Can you work these out from the model? Positions are in its coordinate system, mm. Coordinates: 2 decimals unless noted, no trailing zeros. Loops run counter-clockwise (first coordinate to the right, second up) from the corner with the lowest first, then second, coordinate; pieces in that order, holes last. Notation, with made-up numbers: (82.25, 61) -> (88.25, 61) arc R10 ccw to (88.25, 79) -> close; hole circle Ø2 at (68, 22.25). An arc over 180 degrees is marked (long way). Use one line per item in the form item = value. Start each with the question number.
(1) Imagine slicing it at C-C (y = -24.5). List the corners of the cut face in (x, z) for me.
(2) Imagine slicing it at B-B (z = 8.25). List the corners of the cut face in (x, y) for me.
(3) Imagine slicing it at A-A (x = -3.5). List the corners of the cut face in (y, z) for me.
(4) I need wall thicknesses on line 1 (X direction, y = -22.95, z = 15.5); line 2 (Z direction, x = -44.5, y = -23); line 3 (Z direction, x = -3.5, y = -24.65). Which ranges of each line are inside material? Lowest first, please. Write a range as [from, to].
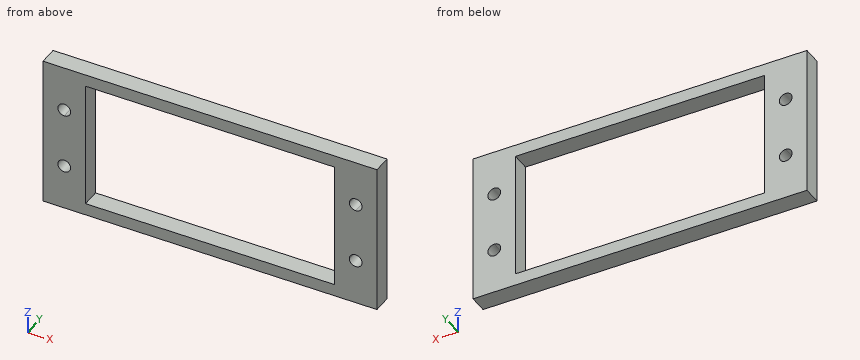
```python
from build123d import *

# Parameters (mm, degrees)
F1_START = 22
F0_W     = 55
F0_H     = 25
F1_DEPTH = 3


with BuildPart() as f1:
    # F0 (on Front) → F1 (new body)
    with BuildSketch(Plane.XZ.offset(F1_START)):
        with Locations((-20.5, 10.5)):
            Rectangle(F0_W, F0_H)
        with BuildLine():
            Line((0, 5.5), (0, 0))
            Line((0, 0), (-41, 0))
            Line((-41, 0), (-41, 5.5))
            Line((-41, 5.5), (-43.45, 5.5))
            ThreePointArc((-43.45, 5.5), (-45.2424621202, 4.7575378798), (-44.5, 6.55))
            Line((-44.5, 6.55), (-44.5, 14.45))
            ThreePointArc((-44.5, 14.45), (-45.2424621202, 16.2424621202), (-43.45, 15.5))
            Line((-43.45, 15.5), (-41, 15.5))
            Line((-41, 15.5), (-41, 21))
            Line((-41, 21), (0, 21))
            Line((0, 21), (0, 15.5))
            Line((0, 15.5), (2.45, 15.5))
            ThreePointArc((2.45, 15.5), (3.5, 16.55), (4.55, 15.5))
            ThreePointArc((4.55, 15.5), (4.2424621202, 14.7575378798), (3.5, 14.45))
            Line((3.5, 14.45), (3.5, 6.55))
            ThreePointArc((3.5, 6.55), (4.2424621202, 6.2424621202), (4.55, 5.5))
            ThreePointArc((4.55, 5.5), (3.5, 4.45), (2.45, 5.5))
            Line((2.45, 5.5), (0, 5.5))
        make_face(mode=Mode.SUBTRACT)
        with BuildLine():
            Line((-43.45, 5.5), (-41, 5.5))
            Line((-41, 5.5), (-41, 15.5))
            Line((-41, 15.5), (-43.45, 15.5))
            ThreePointArc((-43.45, 15.5), (-43.7575378798, 14.7575378798), (-44.5, 14.45))
            Line((-44.5, 14.45), (-44.5, 6.55))
            ThreePointArc((-44.5, 6.55), (-43.7575378798, 6.2424621202), (-43.45, 5.5))
        make_face()
        with BuildLine():
            Line((0, 15.5), (0, 5.5))
            Line((0, 5.5), (2.45, 5.5))
            ThreePointArc((2.45, 5.5), (2.7575378798, 6.2424621202), (3.5, 6.55))
            Line((3.5, 6.55), (3.5, 14.45))
            ThreePointArc((3.5, 14.45), (2.7575378798, 14.7575378798), (2.45, 15.5))
            Line((2.45, 15.5), (0, 15.5))
        make_face()
    extrude(amount=F1_DEPTH)


solid = f1.part
```
Worked out:
q1.outline = (-48, -2) -> (7, -2) -> (7, 23) -> (-48, 23) -> close; hole circle Ø2.1 at (-44.5, 5.5); hole circle Ø2.1 at (-44.5, 15.5); hole (-41, 0) -> (0, 0) -> (0, 21) -> (-41, 21) -> close; hole circle Ø2.1 at (3.5, 5.5); hole circle Ø2.1 at (3.5, 15.5)
q2.outline = (-48, -25) -> (-41, -25) -> (-41, -22) -> (-48, -22) -> close; (0, -25) -> (7, -25) -> (7, -22) -> (0, -22) -> close
q3.outline = (-25, -2) -> (-22, -2) -> (-22, 0) -> (-25, 0) -> close; (-25, 21) -> (-22, 21) -> (-22, 23) -> (-25, 23) -> close
q4.line_1 = [-48, -45.55], [-43.45, -41], [0, 2.45], [4.55, 7]
q4.line_2 = [-2, 4.45], [6.55, 14.45], [16.55, 23]
q4.line_3 = [-2, 0], [21, 23]
